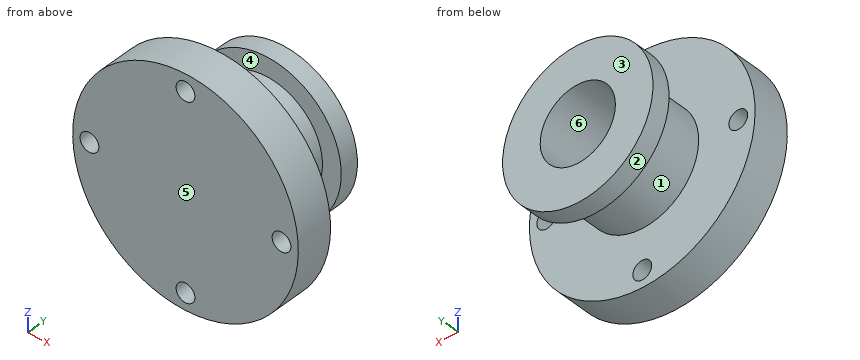
```python
from build123d import *

# Parameters (mm, degrees)
SKETCH5_R          = 25
CUT_EXTRUDE2_DEPTH = 100


with BuildPart() as part:
    # Sketch4 → Revolve2 (revolve)
    with BuildSketch(Plane.XY, mode=Mode.PRIVATE) as revolve2_sk:
        Polygon((0, -251.612903226), (0, -151.612903226), (100, -151.612903226), (100, 48.387096774), (152.822580645, 48.387096774), (200, 48.387096774), (200, -1.612903226), (150, -1.612903226), (150, -151.612903226), (300, -151.612903226), (300, -251.612903226), align=None)
    revolve(revolve2_sk.sketch.rotate(Axis((0, -251.612903226, 0), (0, 1, 0)), 90), axis=Axis((0, -251.612903226, 0), (0, 1, 0)))

    # Sketch5 → Cut-Extrude2 (cut)
    with BuildSketch(Plane(origin=(0, -151.612903226, 0), x_dir=(1, 0, 0), z_dir=(0, 1, 0))):
        with Locations(Location((0, 255.365455535, 0), (0, 0, 270))):
            Circle(SKETCH5_R)
        with Locations(Location((255.365455535, 0, 0), (0, 0, 270))):
            Circle(SKETCH5_R)
        with Locations(Location((0, -255.365455535, 0), (0, 0, 270))):
            Circle(SKETCH5_R)
        with Locations(Location((-255.365455535, 0, 0), (0, 0, 270))):
            Circle(SKETCH5_R)
    extrude(amount=-CUT_EXTRUDE2_DEPTH, mode=Mode.SUBTRACT)


solid = part.part
```
Here's how the part is built. I have some questions about the finished solid (model axes, mm). Face numbers are marked on the shaded views. A direction names the side the tool comes from. Round coordinates to 2 decimals unless told otherwise and drop trailing zeros. Write each loop counter-clockwise with the first axis right and the second up, starting at its lowest first coordinate (ties: lowest second). Pieces come first, ordered by that corner, then holes.
Q1. If we section it at B-B on x = 0: Write out the boundary of the cut face in (y, z), plus the area to 3 significant figures.
Q2. If we section it at C-C on z = 254: Write out the boundary of the cut face in (x, y).
Q3. Please list where these lines run through material, in increasing order: probe 1 along X at (y, z) = (-175, 0); probe 2 along Y at (x, z) = (-55.5, 169.5); probe 3 along Y at (x, z) = (-174, 109).
Q4. If we section it at A-A on z = 0: Write out the boundary of the cut face in (x, y), plus the area to 3 significant figures.
Q5. Will these pins go through, and if not, where does the flat tip stop? P1, Ø1.5, axis at y = -154, z = -94, coming from the +X side; P2, Ø3, axis at x = 114.5, y = -43, coming from the +Z side; P3, Ø1.5, axis at y = -214.5, z = -233.5, coming from the +X side.
Q6. If we section it at D-D on x = -239: Write out the boundary of the cut face in (y, z).
Q7. Which directions (+Z, -Z, +X, -X, +Y, -Y) give clear straight access to the entire face, cutting with the end or side of a thin tool? Please do the marked faces 1, 2 and 3.
Q8. If we mould it in two halves opening along Y, with no side actions, what happens to the marked faces 4, 5 and 6? For each: +Y half, -Y half, draft (parallel to the pull), parting line (faces both ways), or undercut.
Answer below:
1. outline: (-251.61, -300) - (-151.61, -300) - (-151.61, -280.37) - (-251.61, -280.37) - close; (-251.61, -230.37) - (-151.61, -230.37) - (-151.61, -150) - (-1.61, -150) - (-1.61, -200) - (48.39, -200) - (48.39, -100) - (-151.61, -100) - (-151.61, 100) - (48.39, 100) - (48.39, 200) - (-1.61, 200) - (-1.61, 150) - (-151.61, 150) - (-151.61, 230.37) - (-251.61, 230.37) - close; (-251.61, 280.37) - (-151.61, 280.37) - (-151.61, 300) - (-251.61, 300) - close
1. area: 75,000 mm2
2. outline: (-159.64, -251.61) - (-24.96, -251.61) - (-24.96, -151.61) - (-159.64, -151.61) - close; (24.96, -251.61) - (159.64, -251.61) - (159.64, -151.61) - (24.96, -151.61) - close
3. probe 1: x = -300 to -280.37, -230.37 to 230.37, 280.37 to 300
3. probe 2: y = -251.61 to -151.61, -1.61 to 48.39
3. probe 3: y = -251.61 to -151.61
4. outline: (-300, -251.61) - (-280.37, -251.61) - (-280.37, -151.61) - (-300, -151.61) - close; (-230.37, -251.61) - (230.37, -251.61) - (230.37, -151.61) - (150, -151.61) - (150, -1.61) - (200, -1.61) - (200, 48.39) - (100, 48.39) - (100, -151.61) - (-100, -151.61) - (-100, 48.39) - (-200, 48.39) - (-200, -1.61) - (-150, -1.61) - (-150, -151.61) - (-230.37, -151.61) - close; (280.37, -251.61) - (300, -251.61) - (300, -151.61) - (280.37, -151.61) - close
4. area: 75,000 mm2
5. P1: stops at x = 285.14
5. P2: stops at z = 98.65
5. P3: stops at x = 189.28
6. outline: (-251.61, -181.33) - (-151.61, -181.33) - (-151.61, -18.9) - (-251.61, -18.9) - close; (-251.61, 18.9) - (-151.61, 18.9) - (-151.61, 181.33) - (-251.61, 181.33) - close
7. face 1: none
7. face 2: +Y
7. face 3: +Z, -Z, +X, -X, +Y
8. face 4: undercut
8. face 5: -Y half
8. face 6: draft
